Geometry check sheet. Reference: the model listing, model coordinates, mm. Give positions to 0.01 mm unless a question says otherwise; leave off trailing zeros. Write each loop counter-clockwise with the first axis right and the second up, starting at its lowest first coordinate (ties: lowest second). Pieces come first, ordered by that corner, then holes. Notation, with made-up numbers: M -34.5,22.5 L -14.5,22.5 A14 cw -14.5,29.5 Z; hole C -35,12.5 d7. An arc over 180 degrees is marked long. Write each question's results on one line, items separated by ' | '.
```python
from build123d import *

# Parameters (mm, degrees)
SKETCH1_R           = 0.25
BOSS_EXTRUDE1_DEPTH = 10.1
BOSS_EXTRUDE1_DRAFT = -15
SKETCH2_R           = 0.25
BOSS_EXTRUDE2_DEPTH = 10
BOSS_EXTRUDE2_DRAFT = 25
SKETCH3_W           = 14
SKETCH3_H           = 0.2
EXTRUDE_THIN1_DEPTH = 5
SKETCH4_W           = 2.1
SKETCH4_H           = 2.1
BOSS_EXTRUDE3_DEPTH = 0.7
SKETCH5_W           = 2
SKETCH5_H           = 3.8
BOSS_EXTRUDE4_DEPTH = 2.1
SKETCH7_R           = 0.25
BOSS_EXTRUDE5_DEPTH = 9.9
BOSS_EXTRUDE5_DRAFT = -65
SKETCH8_W           = 0.8
SKETCH8_H           = 1.6
BOSS_EXTRUDE6_DEPTH = 0.8
SKETCH9_R           = 0.25
BOSS_EXTRUDE7_DEPTH = 10.2
BOSS_EXTRUDE7_DRAFT = -10


with BuildPart() as part:
    # Sketch1 → Boss-Extrude1 (with draft: the straight prism first)
    with BuildSketch(Plane(origin=(0, 0, 0), x_dir=(1, 0, 0), z_dir=(0, 1, 0))):
        Circle(SKETCH1_R)
    extrude(amount=BOSS_EXTRUDE1_DEPTH)
    # Boss-Extrude1: the draft: its side faces are tilted about the plane it starts from
    boss_extrude1_sides = [part.faces().sort_by_distance(p)[0] for p in [
        (-0.25, 5.05, 0),
    ]]
    draft(boss_extrude1_sides, Plane(origin=(0, 0, 0), x_dir=(1, 0, 0), z_dir=(0, 1, 0)), BOSS_EXTRUDE1_DRAFT)



with BuildPart() as body_2:
    # Sketch2 → Boss-Extrude2 (with draft: the straight prism first)
    with BuildSketch(Plane.XZ):
        with Locations((-3, 0)):
            Circle(SKETCH2_R)
    extrude(amount=-BOSS_EXTRUDE2_DEPTH)
    # Boss-Extrude2: the draft: its side faces are tilted about the plane it starts from
    boss_extrude2_sides = [body_2.faces().sort_by_distance(p)[0] for p in [
        (-3.25, 5, 0),
    ]]
    draft(boss_extrude2_sides, Plane.XZ, BOSS_EXTRUDE2_DRAFT)


with BuildPart() as part_1:
    add(part.part)

    add(body_2.part)  # Extrude-Thin1 merges body 2
    # Sketch3 → Extrude-Thin1 (add)
    with BuildSketch(Plane.XY):
        with Locations((-2.495263261, 0)):
            Rectangle(SKETCH3_W, SKETCH3_H)
        with Locations((-2.495263261, 1)):
            Rectangle(SKETCH3_W, SKETCH3_H)
        with Locations((-2.495263261, 2)):
            Rectangle(SKETCH3_W, SKETCH3_H)
        with Locations((-2.495263261, 3)):
            Rectangle(SKETCH3_W, SKETCH3_H)
        with Locations((-2.495263261, 4)):
            Rectangle(SKETCH3_W, SKETCH3_H)
        with Locations((-2.495263261, 5)):
            Rectangle(SKETCH3_W, SKETCH3_H)
        with Locations((-2.495263261, 6)):
            Rectangle(SKETCH3_W, SKETCH3_H)
        with Locations((-2.495263261, 7)):
            Rectangle(SKETCH3_W, SKETCH3_H)
        with Locations((-2.495263261, 8)):
            Rectangle(SKETCH3_W, SKETCH3_H)
        with Locations((-2.495263261, 9)):
            Rectangle(SKETCH3_W, SKETCH3_H)
        with Locations((-2.495263261, 10)):
            Rectangle(SKETCH3_W, SKETCH3_H)
    extrude(amount=EXTRUDE_THIN1_DEPTH)

    # Sketch4 → Boss-Extrude3 (add)
    with BuildSketch(Plane(origin=(0, 0, 0), x_dir=(1, 0, 0), z_dir=(0, 1, 0))):
        with Locations((-3, 0)):
            Rectangle(SKETCH4_W, SKETCH4_H)
    extrude(amount=-BOSS_EXTRUDE3_DEPTH)

    # Sketch5 → Boss-Extrude4 (add)
    with BuildSketch(Plane.XZ):
        Rectangle(SKETCH5_W, SKETCH5_H)
    extrude(amount=BOSS_EXTRUDE4_DEPTH)


with BuildPart() as boss_extrude5_tool:
    # Sketch7 → Boss-Extrude5 (with draft: the straight prism first)
    with BuildSketch(Plane(origin=(0, 0, 0), x_dir=(1, 0, 0), z_dir=(0, 1, 0))):
        with Locations((-3, 0)):
            Circle(SKETCH7_R)
    extrude(amount=BOSS_EXTRUDE5_DEPTH)
    # Boss-Extrude5: the draft: its side faces are tilted about the plane it starts from
    boss_extrude5_sides = [boss_extrude5_tool.faces().sort_by_distance(p)[0] for p in [
        (-3.25, 4.95, 0),
    ]]
    draft(boss_extrude5_sides, Plane(origin=(0, 0, 0), x_dir=(1, 0, 0), z_dir=(0, 1, 0)), BOSS_EXTRUDE5_DRAFT)


with BuildPart() as part_2:
    add(part_1.part)

    # Boss-Extrude5: add boss_extrude5_tool
    add(boss_extrude5_tool.part)

    # Sketch8 → Boss-Extrude6 (add)
    with BuildSketch(Plane.XZ):
        with Locations((-3, 0)):
            Rectangle(SKETCH8_W, SKETCH8_H)
    extrude(amount=BOSS_EXTRUDE6_DEPTH)


with BuildPart() as boss_extrude7_tool:
    # Sketch9 → Boss-Extrude7 (with draft: the straight prism first)
    with BuildSketch(Plane(origin=(0, 0, 0), x_dir=(1, 0, 0), z_dir=(0, 1, 0))):
        with Locations((-1.5, 0)):
            Circle(SKETCH9_R)
    extrude(amount=BOSS_EXTRUDE7_DEPTH)
    # Boss-Extrude7: the draft: its side faces are tilted about the plane it starts from
    boss_extrude7_sides = [boss_extrude7_tool.faces().sort_by_distance(p)[0] for p in [
        (-1.75, 5.1, 0),
    ]]
    draft(boss_extrude7_sides, Plane(origin=(0, 0, 0), x_dir=(1, 0, 0), z_dir=(0, 1, 0)), BOSS_EXTRUDE7_DRAFT)


with BuildPart() as part_3:
    add(part_2.part)

    # Boss-Extrude7: add boss_extrude7_tool
    add(boss_extrude7_tool.part)


solid = part_3.part
```
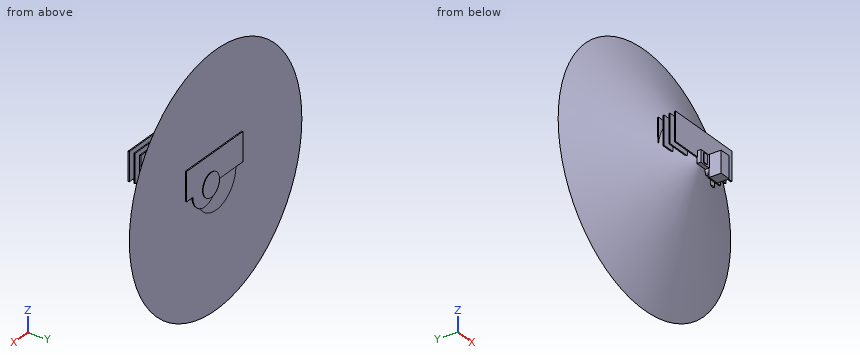
Q1. Section check A-A (y = 7.75). Enter the section's corners in (x, z), then the cut area to 3 significant figures.
Answer key:
outline: C -3,0 d33.74 | area: 894 mm2
Q2. Material ranges on probe 1 along Y at (x, z) = (-3, -2.5); probe 2 along Y at (x, z) = (17.5, -3.5); probe 3 along X at (y, z) = (6.75, 0.5), recorded low to high. Write a range as [from, to].
Answer key:
probe 1: y = [1.05, 10] | probe 2: y = [9.58, 9.9] | probe 3: x = [-17.72, 11.72]
Q3. Depth check by flat-ended pin: P1, Ø6, axis at x = 4.5, z = 6.5, coming from the +Y side; P2, Ø5, axis at x = -4.5, z = -11.5, coming from the -Y side; P3, Ø2, axis at x = 0, y = -1, coming from the -Z side. Enter the tip coordinate at first touch or a pass-through.
Answer key:
P1: stops at y = 10.1 | P2: stops at y = 4.13 | P3: stops at z = -1.9
